Autodesk Inventor part; units mm, degrees
ref_plane "YZ Plane" through (0, 0, 0) normal (1, 0, 0) x (0, 1, 0)
ref_plane "XZ Plane" through (0, 0, 0) normal (0, 1, 0) x (-1, 0, 0)
ref_plane "XY Plane" through (0, 0, 0) normal (0, 0, 1) x (1, 0, 0)
sketch "Sketch1" plane through (0, 0, 0) normal (0, 0, 1) x (1, 0, 0)
  line L0 (-9.1579, 2.8421) -> (-7.1579, 2.8421)
  line L1 (-7.1579, 2.8421) -> (-7.1579, -1.1579)
  line L2 (-7.1579, -1.1579) -> (-9.1579, -1.1579)
  line L3 (-9.1579, -1.1579) -> (-9.1579, 2.8421)
  line L4 (-9.1579, 0.8421) -> (-2.1579, 0.8421)
  line L5 (-2.1579, 0.8421) -> (-2.1579, -1.1579)
  line L6 (-2.1579, -1.1579) -> (-9.1579, -1.1579)
  line L7 (-9.1579, -1.1579) -> (-9.1579, 0.8421)
  line L8 (-2.1579, -1.1579) -> (-4.1579, -1.1579)
  line L9 (-4.1579, -1.1579) -> (-4.1579, 2.8421)
  line L10 (-4.1579, 2.8421) -> (-2.1579, 2.8421)
  line L11 (-2.1579, 2.8421) -> (-2.1579, -1.1579)
  line L12 (-9.1579, 0.8421) -> (-7.1579, 0.8421)
  line L13 (-7.1579, 0.8421) -> (-7.1579, -4.1579)
  line L14 (-7.1579, -4.1579) -> (-9.1579, -4.1579)
  line L15 (-9.1579, -4.1579) -> (-9.1579, 0.8421)
  line L16 (-2.1579, 0.8421) -> (-4.1579, 0.8421)
  line L17 (-4.1579, 0.8421) -> (-4.1579, -4.1579)
  line L18 (-4.1579, -4.1579) -> (-2.1579, -4.1579)
  line L19 (-2.1579, -4.1579) -> (-2.1579, 0.8421)
  point P0 (0, 0)
  dimension "d0" = 2
  dimension "d1" = 2
  dimension "d2" = 3
  dimension "d3" = 3
  dimension "d4" = 2
  dimension "d5" = 2
extrude "Extrusion1" add sketch "Sketch1" along normal blind 25
fillet "Fillet1" radius 1 2 edges at (-5.6579, 0.8421, 25) (-5.6579, -1.1579, 25)
fillet "Fillet2" radius 1 2 edges at (-5.6579, 0.8421, 0) (-5.6579, -1.1579, 0)
properties part number "Cable Sliding Assistor"
Source: CAD feature listing. Evaluate the final solid. Frame: model axes, mm. A direction names the side the tool comes from. Round coordinates to 2 decimals unless told otherwise and drop trailing zeros. Loops run counter-clockwise (first coordinate to the right, second up) from the corner with the lowest first, then second, coordinate; pieces in that order, holes last. Notation, with made-up numbers: (-19.75, -4) - (-4.75, -4) arc R8 cw to (-4.75, 1) - close; hole circle Ø9 at (81, 48.5). An arc over 180 degrees is marked (long way). Write item = value, one per line. Start each with the question number.
Item 1: Section query A-A on y = -1.75. Output: boundary loops of the cut face in (x, z), plus the area to 3 significant figures.
Item 2: Section query C-C on z = 19. Output: boundary loops of the cut face in (x, y), plus the area to 3 significant figures.
Item 3: Reachability of faces 4 (the face through (-5.637, 0.542, 0.285)), 5 (the face through (-6, 0.842, 12)), 6 (the face through (-5.637, 0.557, 24.699)), 7 (the face through (-6, -1.158, 12)), 8 (the face through (-5.68, -0.86, 0.29)) from +Z, -Z, +X, -X, +Y, -Y: full face, straight path, thin tool, end or side. Return the list, or none.
Item 4: First-contact query: pin 1 Ø2 at (x, z) = (-5.5, 10) entering from +Y. Flat tip, straight axial feed; report the tip coordinate or a pass-through.
Item 5: Mould query, pull axis X, two halves, no side actions, for faces 1 (the face through (-4, -1, 0)), 2 (the face through (-2.158, -1, 12)), 3 (the face through (-5.68, -0.87, 24.7)). Classes: released by +X, released by -X, zero draft, split by the parting line, or undercut.
Item 6: Material intervals for line 1 (X direction, y = -1.75, z = 23); line 2 (Y direction, x = -5.25, z = 11.75); line 3 (Z direction, x = -5.25, y = 0), sorted ascending.
Results list:
q1.outline = (-9.16, 0) - (-7.16, 0) - (-7.16, 25) - (-9.16, 25) - close; (-4.16, 0) - (-2.16, 0) - (-2.16, 25) - (-4.16, 25) - close
q1.area = 100 mm²
q2.outline = (-9.16, -4.16) - (-7.16, -4.16) - (-7.16, -1.16) - (-4.16, -1.16) - (-4.16, -4.16) - (-2.16, -4.16) - (-2.16, 2.84) - (-4.16, 2.84) - (-4.16, 0.84) - (-7.16, 0.84) - (-7.16, 2.84) - (-9.16, 2.84) - close
q2.area = 34.0 mm²
q3.face_4 = -Z, +Y
q3.face_5 = +Z, -Z, +Y
q3.face_6 = +Z, +Y
q3.face_7 = +Z, -Z, -Y
q3.face_8 = -Z, -Y
q4.pin_1 = 0.84
q5.face_1 = zero draft
q5.face_2 = released by +X
q5.face_3 = undercut
q6.line_1 = -9.16 to -7.16, -4.16 to -2.16
q6.line_2 = -1.16 to 0.84
q6.line_3 = 0.01 to 24.99
